```python
from build123d import *

# Parameters (mm, degrees)
ESBO_O1_W             = 8.35
ESBO_O1_H             = 5
CORTE_EXTRUS_O1_DEPTH = 3
ESBO_O4_R             = 1
CORTE_EXTRUS_O2_DEPTH = 10


with BuildPart() as part:
    # Esboço1 → Revolução1 (revolve)
    with BuildSketch(Plane.XY):
        with Locations((-5.825, 2.5)):
            Rectangle(ESBO_O1_W, ESBO_O1_H)
    revolve(axis=Axis((0, 0, 0), (0, 1, 0)))

    # Esboço3 → Corte-extrusão1 (cut)
    with BuildSketch(Plane.XZ):
        Polygon((3.175426481, 0), (1.58771324, 2.75), (-1.58771324, 2.75), (-3.175426481, 0), (-1.58771324, -2.75), (1.58771324, -2.75), align=None)
    extrude(amount=-CORTE_EXTRUS_O1_DEPTH, mode=Mode.SUBTRACT)

    # Esboço4 → Corte-extrusão2 (cut)
    with BuildSketch(Plane(origin=(0, 5, 0), x_dir=(1, 0, 0), z_dir=(0, 1, 0))):
        with Locations((0, 10)):
            Circle(ESBO_O4_R)
        with Locations((3.090169944, 9.510565163)):
            Circle(ESBO_O4_R)
        with Locations((5.877852523, 8.090169944)):
            Circle(ESBO_O4_R)
        with Locations((8.090169944, 5.877852523)):
            Circle(ESBO_O4_R)
        with Locations((9.510565163, 3.090169944)):
            Circle(ESBO_O4_R)
        with Locations((10, 0)):
            Circle(ESBO_O4_R)
        with Locations((9.510565163, -3.090169944)):
            Circle(ESBO_O4_R)
        with Locations((8.090169944, -5.877852523)):
            Circle(ESBO_O4_R)
        with Locations((5.877852523, -8.090169944)):
            Circle(ESBO_O4_R)
        with Locations((3.090169944, -9.510565163)):
            Circle(ESBO_O4_R)
        with Locations((0, -10)):
            Circle(ESBO_O4_R)
        with Locations((-3.090169944, -9.510565163)):
            Circle(ESBO_O4_R)
        with Locations((-5.877852523, -8.090169944)):
            Circle(ESBO_O4_R)
        with Locations((-8.090169944, -5.877852523)):
            Circle(ESBO_O4_R)
        with Locations((-9.510565163, -3.090169944)):
            Circle(ESBO_O4_R)
        with Locations((-10, 0)):
            Circle(ESBO_O4_R)
        with Locations((-9.510565163, 3.090169944)):
            Circle(ESBO_O4_R)
        with Locations((-8.090169944, 5.877852523)):
            Circle(ESBO_O4_R)
        with Locations((-5.877852523, 8.090169944)):
            Circle(ESBO_O4_R)
        with Locations((-3.090169944, 9.510565163)):
            Circle(ESBO_O4_R)
    extrude(amount=-CORTE_EXTRUS_O2_DEPTH, mode=Mode.SUBTRACT)


solid = part.part
```
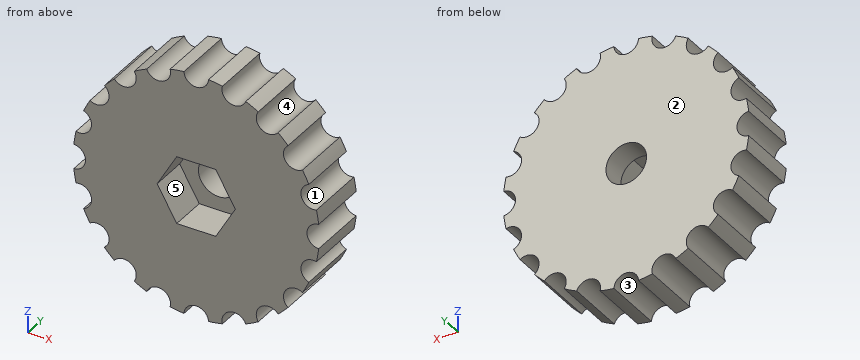
Input: part model. Units: mm. Frame: model coordinates. Face numbers are marked on the shaded views. A direction names the side the tool comes from. Give positions to 0.01 mm unless a question says otherwise; leave off trailing zeros. Write each loop counter-clockwise with the first axis right and the second up, starting at its lowest first coordinate (ties: lowest second). Pieces come first, ordered by that corner, then holes. Notation, with made-up numbers: (-7, -17.75) - (13, -17.75) arc R15 ccw to (13, 5.25) - close; hole circle Ø5 at (-37.75, 32). An arc over 180 degrees is marked (long way). Write item = value, one per line. Start each with the question number.
1. Section query D-D, the plane z = 8. Output: boundary loops of the cut face in (x, y), then the cut area to 3 significant figures.
2. Ray query, L1, parallel to Z at x = 0, y = 4; L2, parallel to X at y = 3.65, z = -3; L3, parallel to Z at x = -8, y = 1.25. Return the intervals inside material, ascending.
3. Access query for the marked faces 4 and 5. Directions: +Z, -Z, +X, -X, +Y, -Y. A direction counts if a zero-diameter tool reaches every point of the face in a straight line with its end or side. Return the directions, or none.
4. First-contact query: pin 1 Ø2 at (x, z) = (0, 0) entering from -Y; pin 2 Ø1.5 at (x, y) = (0, 1) entering from -Z; pin 3 Ø1 at (y, z) = (4, 5) entering from -X; pin 4 Ø3 at (x, y) = (-6.5, 1) entering from +Z. Flat tips, straight axial feed; report the tip coordinate or a pass-through.
5. Mould query, pull axis Z, two halves, no side actions, for the marked faces 1, 2 and 3. Classes: released by +Z, released by -Z, zero draft, split by the parting line, or undercut.
6. Section query A-A, the plane x = 0. Output: boundary loops of the cut face in (y, z), then the cut area to 3 significant figures.
7. Section query B-B, the plane z = 0.5. Output: boundary loops of the cut face in (x, y), then the cut area to 3 significant figures.
8. Section query C-C, the plane z = 4.5. Output: boundary loops of the cut face in (x, y), then the cut area to 3 significant figures.
Check sheet entries:
q1.outline = (-4.88, 0) - (4.88, 0) - (4.88, 5) - (-4.88, 5) - close
q1.area = 48.8 mm2
q2.L1 = -9 to -1.65, 1.65 to 9
q2.L2 = -8.51 to 8.51
q2.L3 = -4.88 to 4.88
q3.face_4 = +Y, -Y
q3.face_5 = -Y
q4.pin_1 = through
q4.pin_2 = -9.34
q4.pin_3 = -8.93
q4.pin_4 = 8.66
q5.face_1 = undercut
q5.face_2 = zero draft
q5.face_3 = released by -Z
q6.outline = (0, -9) - (5, -9) - (5, -1.65) - (3, -1.65) - (3, -2.75) - (0, -2.75) - close; (0, 2.75) - (3, 2.75) - (3, 1.65) - (5, 1.65) - (5, 9) - (0, 9) - close
q6.area = 66.9 mm2
q7.outline = (-9.13, 0) - (-2.89, 0) - (-2.89, 3) - (-1.57, 3) - (-1.57, 5) - (-9.13, 5) - close; (1.57, 3) - (2.89, 3) - (2.89, 0) - (9.13, 0) - (9.13, 5) - (1.57, 5) - close
q7.area = 67.7 mm2
q8.outline = (-8.93, 0) - (8.93, 0) - (8.93, 5) - (-8.93, 5) - close
q8.area = 89.3 mm2
